Here's the drawing with two shaded views (mm, measured from the low corner). I have some questions. Coordinates: 2 decimals unless noted, no trailing zeros. Write each loop counter-clockwise with the first axis right and the second up, starting at its lowest first coordinate (ties: lowest second). Pieces come first, ordered by that corner, then holes. Notation, with made-up numbers: M 39.25,69 L 91.25,69 A21 ccw 91.25,94 Z; hole C 44.5,-22 d11. An arc over 180 degrees is marked long. Use one line per item in the form item = value. Start each with the question number.
1. I want a section at D-D, the plane y = 244. List the corners of the cut face in (x, z) for me.
2. I'm going to push flat-ended pins straight in: pin 1 Ø0.9 at (x, z) = (184.5, 2) entering from +Y; pin 2 Ø0.9 at (y, z) = (208.5, 1) entering from -X; pin 3 Ø1.5 at (y, z) = (219.5, 1) entering from +X. Where does each tip first touch, or does it pass through?
3. Please list where these lines run through material, in increasing order: line 1 along Y through (x, z) = (150.5, 0.7); line 2 along X through (y, z) = (205.5, 0.5); line 3 along Y through (x, z) = (83, 0.35). Write a range as [from, to].
4. I want a section at C-C, the plane x = 186. List the corners of the cut face in (y, z) for me.
5. I want a section at A-A, the plane x = 106. List the corners of the cut face in (y, z) for me, plus the area to 3 significant figures.
6. I want a section at B-B, the plane y = 158.5. List the corners of the cut face in (x, z) for me, plus the area to 3 significant figures.
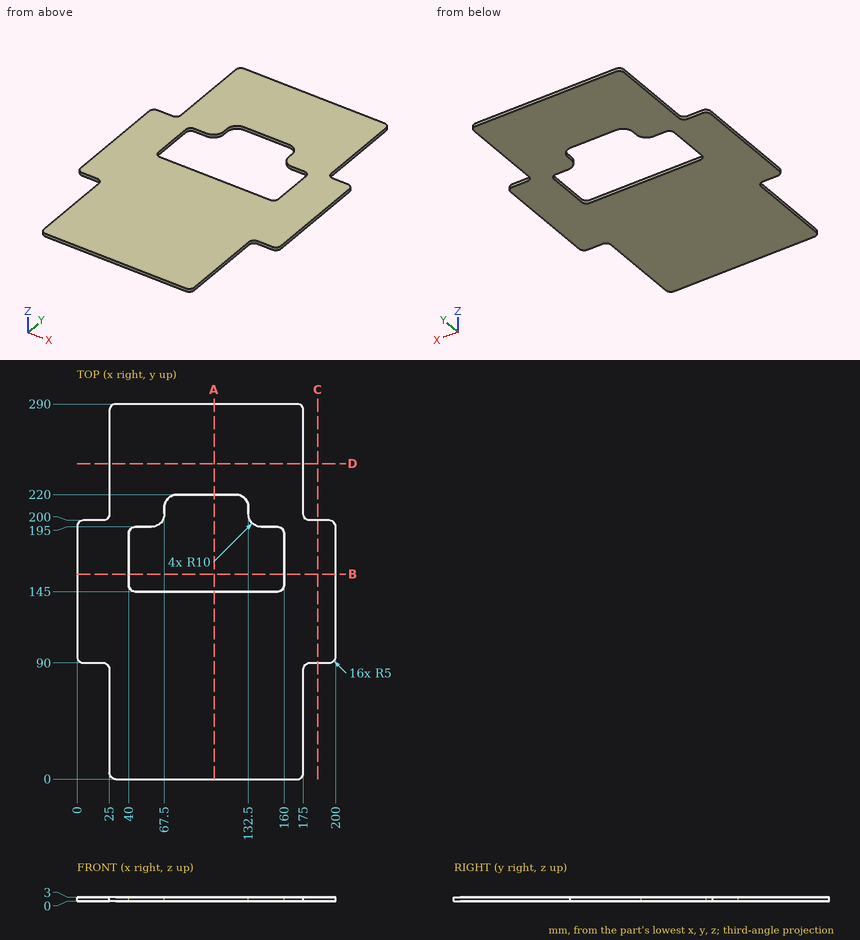
Answer list:
q1.outline = M 25,0 L 175,0 L 175,3 L 25,3 Z
q2.pin_1 = 200
q2.pin_2 = 25
q2.pin_3 = 175
q3.line_1 = [0, 145], [195, 290]
q3.line_2 = [25, 67.5], [132.5, 175]
q3.line_3 = [0, 145], [220, 290]
q4.outline = M 90,0 L 200,0 L 200,3 L 90,3 Z
q5.outline = M 0,0 L 145,0 L 145,3 L 0,3 Z; M 220,0 L 290,0 L 290,3 L 220,3 Z
q5.area = 645 mm²
q6.outline = M 0,0 L 40,0 L 40,3 L 0,3 Z; M 160,0 L 200,0 L 200,3 L 160,3 Z
q6.area = 240 mm²
